Can you work these out from the model? Positions are in its coordinate system, mm. Coordinates: 2 decimals unless noted, no trailing zeros. Order: outer loops, then holes, each group sorted by start corner. A loop starts at its lowest first (then second) coordinate and runs counter-clockwise, first axis right, second up. Notation, with made-up numbers: (52, 84.25) -> (65, 84.25) arc R29 cw to (65, 111.25) -> close; hole circle Ø3 at (-3.5, -5). An arc over 180 degrees is marked (long way). Answer as a JSON object with one key per item and string values. Group by question number.
(1) I want a section at B-B, the plane x = 47.5. List the corners of the cut face in (y, z) for me.
(2) For pin 1 (0.9 mm diameter, centred on y = 1.5, z = -93, fed in from +X); pin 2 (1 mm diameter, centred on y = 2, z = -65, fed in from -X); pin 3 (0.9 mm diameter, centred on x = 2, y = 1, fed in from -Z), each with a flat end and sliding along its axis, tell me the tip position at first contact or that it passes through.
(3) I need wall thicknesses on line 1 (Z direction, x = 18, y = 2.05); line 2 (X direction, y = 1.4, z = -9); line 3 (Z direction, x = 53, y = 0.9). Which ranges of each line are inside material? Lowest first, please.
(4) I want a section at A-A, the plane z = 3. List the corners of the cut face in (x, y) for me.
from build123d import *

# Parameters (mm, degrees)
BOSS_EXTRU_1_DEPTH = 3


with BuildPart() as part:
    # Esquisse1 → Boss.-Extru.1 (new body)
    with BuildSketch(Plane(origin=(0, 0, 0), x_dir=(1, 0, 0), z_dir=(0, 1, 0))):
        Polygon((3, 0), (0, 0), (10, -30), (16, -30), (16, -27), (24, -27), (24, -30), (36, -30), (36, -27), (44, -27), (44, -30), (56, -30), (56, -27), (64, -27), (64, -30), (76, -30), (76, -27), (84, -27), (84, -30), (90, -30), (100, 0), (97, 0), (97, 14.2), (100, 14.2), (100, 22.8), (97, 22.8), (97, 34.2), (100, 34.2), (100, 42.8), (97, 42.8), (97, 54.2), (100, 54.2), (100, 62.8), (97, 62.8), (97, 74.2), (100, 74.2), (100, 82.8), (97, 82.8), (97, 95), (94, 95), (94, 92), (86, 92), (86, 95), (74, 95), (74, 92), (66, 92), (66, 95), (54, 95), (54, 92), (46, 92), (46, 95), (34, 95), (34, 92), (26, 92), (26, 95), (14, 95), (14, 92), (6, 92), (6, 95), (3, 95), (3, 82.8), (0, 82.8), (0, 74.2), (3, 74.2), (3, 62.8), (0, 62.8), (0, 54.2), (3, 54.2), (3, 42.8), (0, 42.8), (0, 34.2), (3, 34.2), (3, 22.8), (0, 22.8), (0, 14.2), (3, 14.2), align=None)
    extrude(amount=BOSS_EXTRU_1_DEPTH)


solid = part.part
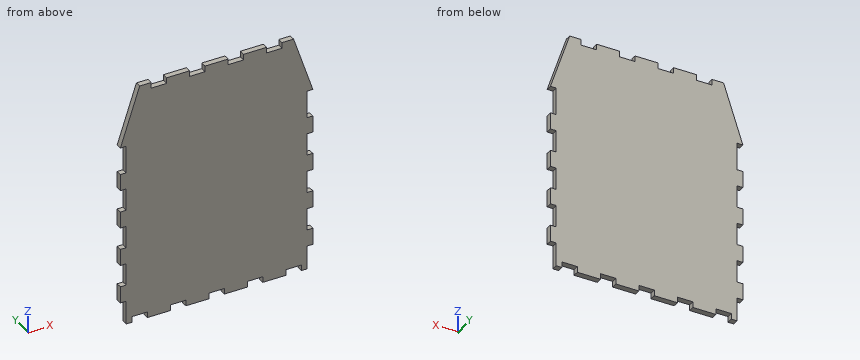
Computed values:
{
 "1": {"outline": "(0, -92) -> (3, -92) -> (3, 30) -> (0, 30) -> close"},
 "2": {"pin 1": "stops at x = 97", "pin 2": "stops at x = 3", "pin 3": "stops at z = -82.8"},
 "3": {"line 1": "z = -95 to 27", "line 2": "x = 3 to 97", "line 3": "z = -92 to 30"},
 "4": {"outline": "(1, 0) -> (99, 0) -> (99, 3) -> (1, 3) -> close"}
}
